Verification items for this drawing (mm, ordinates from the low corner). Coordinates: 2 decimals unless noted, no trailing zeros. Write each loop counter-clockwise with the first axis right and the second up, starting at its lowest first coordinate (ties: lowest second). Pieces come first, ordered by that corner, then holes. Notation, with made-up numbers: (61.5, -9.75) -> (77.5, -9.75) arc R29 ccw to (77.5, 22.25) -> close; hole circle Ø11 at (50, -38). An arc over 180 degrees is marked (long way). Answer as CSV lines item,"result".
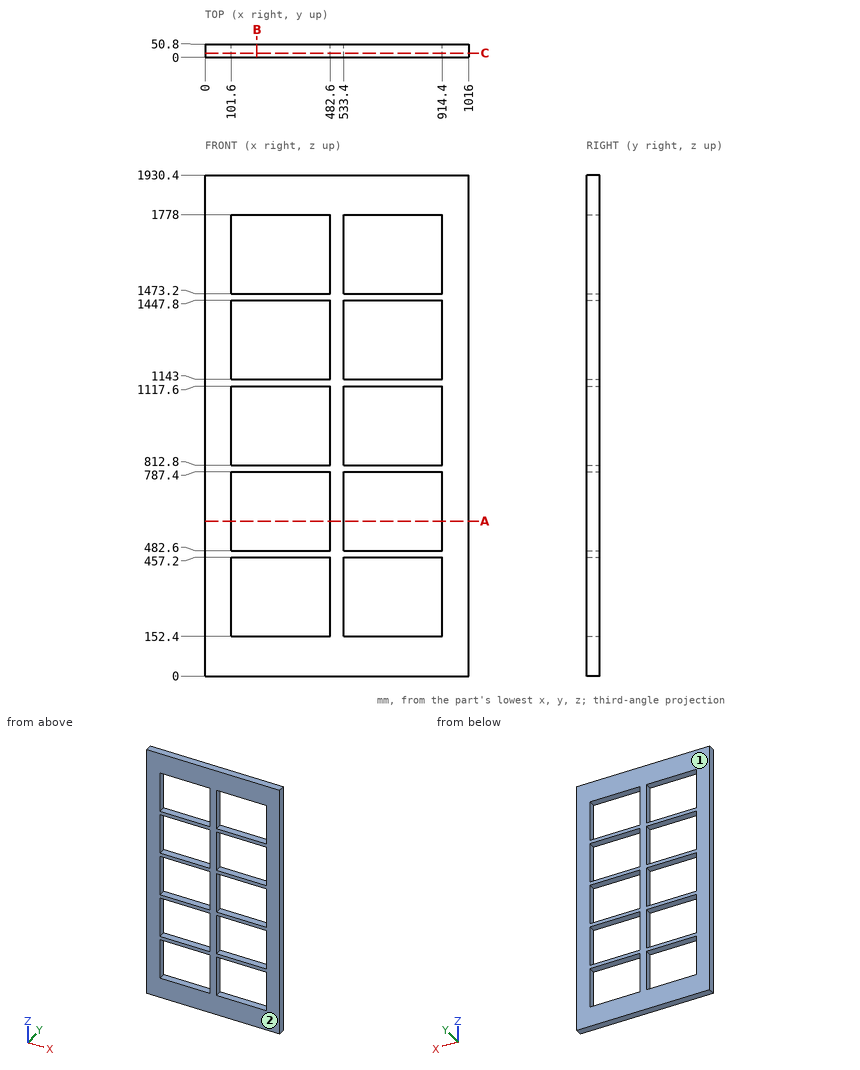
Item 1: Cross-section at C-C, the plane y = 16. Count the separate pieces of the cut face and the enclosed holes in it, plus the area to 3 significant figures.
Responses:
separate pieces,"1"
enclosed holes,"10"
area,"800,000 mm2"
Item 2: Cross-section at A-A, the plane z = 597. Record the cut outline in (x, y).
Responses:
outline,"(0, 0) -> (101.6, 0) -> (101.6, 50.8) -> (0, 50.8) -> close; (482.6, 0) -> (533.4, 0) -> (533.4, 50.8) -> (482.6, 50.8) -> close; (914.4, 0) -> (1016, 0) -> (1016, 50.8) -> (914.4, 50.8) -> close"
Item 3: Thickness scan on probe 1 along Z at (x, y) = (832, 47); probe 2 along X at (y, z) = (20, 400.5). Record the ranges inside material, lowest first.
Responses:
probe 1,"z = 0 to 152.4, 457.2 to 482.6, 787.4 to 812.8, 1117.6 to 1143, 1447.8 to 1473.2, 1778 to 1930.4"
probe 2,"x = 0 to 101.6, 482.6 to 533.4, 914.4 to 1016"
Item 4: Cross-section at B-B, the plane x = 199.5. Record the cut outline in (y, z), plus the area to 3 significant figures.
Responses:
outline,"(0, 0) -> (50.8, 0) -> (50.8, 152.4) -> (0, 152.4) -> close; (0, 457.2) -> (50.8, 457.2) -> (50.8, 482.6) -> (0, 482.6) -> close; (0, 787.4) -> (50.8, 787.4) -> (50.8, 812.8) -> (0, 812.8) -> close; (0, 1117.6) -> (50.8, 1117.6) -> (50.8, 1143) -> (0, 1143) -> close; (0, 1447.8) -> (50.8, 1447.8) -> (50.8, 1473.2) -> (0, 1473.2) -> close; (0, 1778) -> (50.8, 1778) -> (50.8, 1930.4) -> (0, 1930.4) -> close"
area,"20,600 mm2"
Item 5: Release check for a two-part mould opening along Y. For the marked faces 1 and 2 record: +Y half, -Y half, draft (parallel to the pull), parting line (faces both ways), or undercut.
Responses:
face 1,"+Y half"
face 2,"-Y half"
